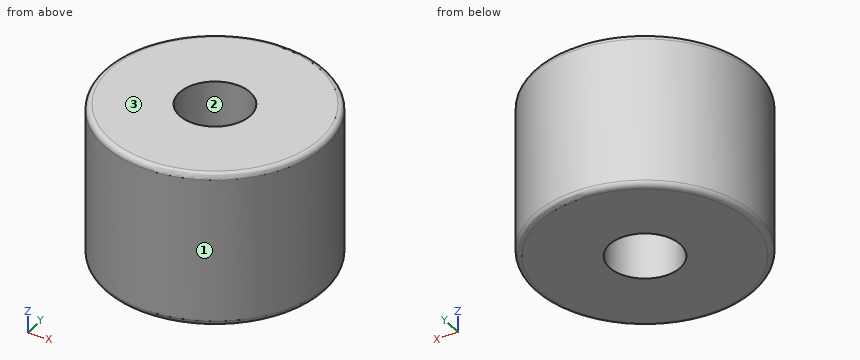
from build123d import *

# Parameters (mm, degrees)
ESQUISSE1_R        = 5
ESQUISSE1_R_2      = 1.6
BOSS_EXTRU_1_DEPTH = 7
CONG_1_R           = 0.25
CONG_2_R           = 0.25


with BuildPart() as part:
    # Esquisse1 → Boss.-Extru.1 (new body)
    with BuildSketch(Plane.XY):
        Circle(ESQUISSE1_R)
        Circle(ESQUISSE1_R_2, mode=Mode.SUBTRACT)
    extrude(amount=BOSS_EXTRU_1_DEPTH)

    # Congé1
    cong_1_edges = [part.edges().sort_by_distance(p)[0] for p in [
        (-5, 0, 7),
    ]]
    fillet(cong_1_edges, radius=CONG_1_R)

    # Congé2
    cong_2_edges = [part.edges().sort_by_distance(p)[0] for p in [
        (-5, 0, 0),
    ]]
    fillet(cong_2_edges, radius=CONG_2_R)


solid = part.part
Read the model definition and answer for the solid it produces. Units are mm, in the model's axes. Face numbers are marked on the shaded views. Give positions to 0.01 mm unless a question says otherwise; leave off trailing zeros. Loops run counter-clockwise (first coordinate to the right, second up) from the corner with the lowest first, then second, coordinate; pieces in that order, holes last. Notation, with made-up numbers: (69, 51.5) -> (120, 51.5) arc R27 ccw to (120, 72.5) -> close; hole circle Ø9 at (64, 77.5). An arc over 180 degrees is marked (long way). Answer as CSV lines item,"result".
Item 1: Each of these flat-tipped pins is pushed along its axis until it touches: pin 1 (2 mm diameter, centred on x = 2.5, z = 3.5, fed in from +Y); pin 2 (3 mm diameter, centred on x = -3.5, z = 4.5, fed in from +Y); pin 3 (1 mm diameter, centred on x = -4, y = 3.5, fed in from +Z). Where does it stop, or does it pass through?
Returned:
pin 1,"stops at y = 4.77"
pin 2,"stops at y = 4.58"
pin 3,"stops at z = 6.99"
Item 2: Consider line 1 (Y direction, x = 0, z = 2.25); line 2 (X direction, y = -0.5, z = 1); line 3 (Y direction, x = -1.25, z = 2.25). Determine where each line is inside the solid, lowest interval first. Write a range as [from, to].
Returned:
line 1,"y = [-5, -1.6], [1.6, 5]"
line 2,"x = [-4.97, -1.52], [1.52, 4.97]"
line 3,"y = [-4.84, -1], [1, 4.84]"
Item 3: Find section C-C on z = 4.25. Give the vertices of the cut face in (x, y).
Returned:
outline,"circle Ø10 at (0, 0); hole circle Ø3.2 at (0, 0)"
Item 4: Determine the mould class of the marked faces 1, 2 and 3 for opening direction Y: +Y half, -Y half, draft (parallel to the pull), parting line (faces both ways), or undercut.
Returned:
face 1,"parting line"
face 2,"undercut"
face 3,"draft"
Item 5: Find section A-A on y = 0. Give the vertices of the cut face in (x, z).
Returned:
outline,"(-5, 0.25) arc R0.25 ccw to (-4.75, 0) -> (-1.6, 0) -> (-1.6, 7) -> (-4.75, 7) arc R0.25 ccw to (-5, 6.75) -> close; (1.6, 0) -> (4.75, 0) arc R0.25 ccw to (5, 0.25) -> (5, 6.75) arc R0.25 ccw to (4.75, 7) -> (1.6, 7) -> close"
